The listing builds one solid part. Answer for the finished solid, in the listing's coordinates (mm). A direction names the side the tool comes from. Coordinates: 2 decimals unless noted, no trailing zeros. Order: outer loops, then holes, each group sorted by start corner. A loop starts at its lowest first (then second) coordinate and runs counter-clockwise, first axis right, second up.
from build123d import *

# Parameters (mm, degrees)
F0_W     = 52.765369
F0_H     = 36.238667
F1_DEPTH = 23.368
F2_R     = 12.639817
F3_DEPTH = 10.414
F5_D     = 16.51


with BuildPart() as f1:
    # F0 (on Front) → F1 (new body)
    with BuildSketch(Plane.XZ):
        with Locations((26.382684, 18.119333)):
            Rectangle(F0_W, F0_H)
    extrude(amount=F1_DEPTH)

    # F2 (on face) → F3 (join)
    with BuildSketch(Plane.XZ.offset(23.368)):
        with Locations((25.712097, 18.603459)):
            Circle(F2_R)
    extrude(amount=F3_DEPTH)

    # F5 (through all)
    with Locations(Plane.XZ.offset(33.782)):
        with Locations((25.712097, 18.603459)):
            Hole(F5_D / 2)


solid = f1.part
1) Determine the mould class of faces 1 (the face through (26, -12, 36.239)), 2 (the face through (26, -12, 0)), 3 (the face through (26, 0, 10)), 4 (the face through (26.787, -16.655, 26.788)) for opening direction Z: released by +Z, released by -Z, zero draft, split by the parting line, or undercut.
2) Section D-D (z = 5) is taken. Give the vertices of the cut face in (x, y).
3) A tool of negligible diameter and unlimited length cuts with its end or side. For faces 5 (the face through (22.972, -28.502, 6.264)), 6 (the face through (28, -33.782, 10)), from which of +Z, -Z, +X, -X, +Y, -Y can it reach the whole face along a straight path? Write none if from no direction.
4) Consider L1, parallel to Y at x = 45.5, z = 2.5; L2, parallel to X at y = -26, z = 14; L3, parallel to Z at x = 18.5, y = -15. Determine where each line is inside the solid, lowest interval first.
5) Each of these flat-tipped pins is pushed along its axis until it touches: P1, Ø10, axis at x = 25.5, y = -29, coming from the +Z side; P2, Ø3, axis at y = -26, z = 8, coming from the -X side; P3, Ø10, axis at y = -30, z = 9, coming from the -X side. Where does it stop, or does it pass through?
6) Section B-B (x = 29) is taken. Give the vertices of the cut face in (y, z).
7) Section C-C (x = 35) is taken. Give the vertices of the cut face in (y, z), then the cut area to 3 significant figures.
8) Section A-A (z = 22.5) is taken. Give the vertices of the cut face in (x, y).
Filled sheet:
1. face 1: released by +Z
1. face 2: released by -Z
1. face 3: zero draft
1. face 4: undercut
2. outline: (0, -23.37) - (52.77, -23.37) - (52.77, 0) - (0, 0) - close
3. face 5: -Y
3. face 6: +Z, -Z, +X, -X, -Y
4. L1: y = -23.37 to 0
4. L2: x = 13.94 to 18.86, 32.56 to 37.48
4. L3: z = 0 to 14.59, 22.62 to 36.24
5. P1: stops at z = 31.24
5. P2: stops at x = 16.94
5. P3: stops at x = 13.94
6. outline: (-33.78, 6.4) - (-23.37, 6.4) - (-23.37, 0) - (0, 0) - (0, 11.03) - (-33.78, 11.03) - close; (-33.78, 26.18) - (0, 26.18) - (0, 36.24) - (-23.37, 36.24) - (-23.37, 30.81) - (-33.78, 30.81) - close
7. outline: (-33.78, 10.03) - (-23.37, 10.03) - (-23.37, 0) - (0, 0) - (0, 36.24) - (-23.37, 36.24) - (-23.37, 27.18) - (-33.78, 27.18) - close
7. area: 1,030 mm2
8. outline: (0, -23.37) - (13.69, -23.37) - (13.69, -33.78) - (18.43, -33.78) - (18.43, 0) - (0, 0) - close; (32.99, -33.78) - (37.74, -33.78) - (37.74, -23.37) - (52.77, -23.37) - (52.77, 0) - (32.99, 0) - close
